Autodesk Inventor part; units mm, degrees
ref_plane "YZ Plane" through (0, 0, 0) normal (1, 0, 0) x (0, 1, 0)
ref_plane "XZ Plane" through (0, 0, 0) normal (0, 1, 0) x (-1, 0, 0)
ref_plane "XY Plane" through (0, 0, 0) normal (0, 0, 1) x (1, 0, 0)
sketch "Sketch1" plane through (0, 0, 0) normal (0, 0, 1) x (1, 0, 0)
  circle A0 centre (0, 0) radius 2.4
  arc A1 (21.7188, -1.8155) -> (18.6153, 2.0815) centre (20, 0) ccw
  arc A2 (3.5202, 3.5508) -> (-2.6562, -4.2361) centre (0, 0) ccw
  circle A3 centre (20, 0) radius 0.925
  arc A4 (-2.6562, -4.2361) -> (21.7188, -1.8155) centre (7.9688, 12.7082) ccw
  arc A5 (3.5202, 3.5508) -> (18.6153, 2.0815) centre (11.9688, 12.0727) ccw
  dimension "d0" = 4.8
  dimension "d3" = 2.5
  dimension "d6" = 5
  dimension "d7" = 20
  dimension "d8" = 1.85
  dimension "d9" = 20
  dimension "d10" = 12
extrude "Extrusion1" add sketch "Sketch1" along normal blind 6.2
properties part number "slider_link_p4"
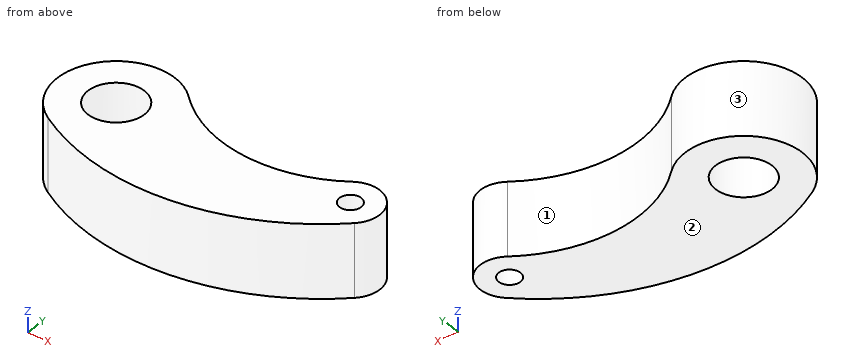
The listing builds one solid part. Answer for the finished solid, in the listing's coordinates (mm). Face numbers are marked on the shaded views. Coordinates: 2 decimals unless noted, no trailing zeros. Loops run counter-clockwise (first coordinate to the right, second up) from the corner with the lowest first, then second, coordinate; pieces in that order, holes last. Notation, with made-up numbers: (-14, 84) -> (22, 84) arc R18 ccw to (22, 95) -> close; hole circle Ø6 at (11, 89). An arc over 180 degrees is marked (long way). Return JSON: item names as keys, results as strings. Group by question number.
(1) Find the intervals of material crossed by probe 1 along Y at (x, z) = (0, 3.5); probe 2 along X at (y, z) = (-1.5, 0.75); probe 3 along Y at (x, z) = (20, 2.75) (3 decimals), in increasing order. Write a range as from..to.
(2) A cutting plane is placed at C-C on y = -1.25. Write down the section's boundary in (x, z), and give its area (3 significant figures).
(3) Determine the mould class of the marked faces 1, 2 and 3 for opening direction X: released by +X, released by -X, zero draft, split by the parting line, or undercut.
(4) A cutting plane is placed at A-A on x = 20. Write down the section's boundary in (y, z) (3 decimals), and give its area (3 significant figures).
(5) A cutting plane is placed at B-B on y = 0.5. Write down the section's boundary in (x, z), and give its area (3 significant figures).
(6) A cutting plane is placed at D-D on z = 4.5. Count the separate pieces of the cut face and the enclosed holes in it, and give its area (3 significant figures).
The answers:
{
 "1": {"probe 1": "y = -5.64..-2.4, 2.4..5", "probe 2": "x = -4.77..-1.87, 1.87..22", "probe 3": "y = -3.268..-0.925, 0.925..2.5"},
 "2": {"outline": "(-4.84, 0) -> (-2.05, 0) -> (-2.05, 6.2) -> (-4.84, 6.2) -> close; (2.05, 0) -> (22.17, 0) -> (22.17, 6.2) -> (2.05, 6.2) -> close", "area": "142 mm^2"},
 "3": {"face 1": "undercut", "face 2": "zero draft", "face 3": "split by the parting line"},
 "4": {"outline": "(-3.268, 0) -> (-0.925, 0) -> (-0.925, 6.2) -> (-3.268, 6.2) -> close; (0.925, 0) -> (2.5, 0) -> (2.5, 6.2) -> (0.925, 6.2) -> close", "area": "24.3 mm^2"},
 "5": {"outline": "(-4.97, 0) -> (-2.35, 0) -> (-2.35, 6.2) -> (-4.97, 6.2) -> close; (2.35, 0) -> (8.79, 0) -> (8.79, 6.2) -> (2.35, 6.2) -> close; (15.14, 0) -> (19.22, 0) -> (19.22, 6.2) -> (15.14, 6.2) -> close; (20.78, 0) -> (22.45, 0) -> (22.45, 6.2) -> (20.78, 6.2) -> close", "area": "91.9 mm^2"},
 "6": {"separate pieces": "1", "enclosed holes": "2", "area": "189 mm^2"}
}
